from build123d import *

# Parameters (mm, degrees)
SKETCH1_W             = 152.4
SKETCH1_H             = 152.4
SKETCH1_W_2           = 127
SKETCH1_H_2           = 127
BOSS_EXTRUDE1_DEPTH   = 3.175
F_8_CLEARANCE_HOLE2_D = 4.4958
LPATTERN1_COUNT       = 2
LPATTERN1_PITCH       = 139.7
LPATTERN1_COUNT_DIR2  = 2
LPATTERN1_PITCH_DIR2  = 139.7


with BuildPart() as part:
    # Sketch1 → Boss-Extrude1 (new body)
    with BuildSketch(Plane.XY):
        with Locations((38.331291391, -35.471688742)):
            Rectangle(SKETCH1_W, SKETCH1_H)
        with Locations((38.331291391, -35.471688742)):
            Rectangle(SKETCH1_W_2, SKETCH1_H_2, mode=Mode.SUBTRACT)
    extrude(amount=BOSS_EXTRUDE1_DEPTH)

    # #8 Clearance Hole2 (through all)
    with Locations(Plane.XY.offset(3.175)):
        with Locations((-31.616116629, 34.273559139)):
            f_8_clearance_hole2 = Hole(F_8_CLEARANCE_HOLE2_D / 2)

    # LPattern1: 8 Clearance Hole2 2 × 2
    with Locations(*[(i * LPATTERN1_PITCH, -j * LPATTERN1_PITCH_DIR2, 0) for i in range(LPATTERN1_COUNT) for j in range(LPATTERN1_COUNT_DIR2) if (i, j) != (0, 0)]):
        add(f_8_clearance_hole2, mode=Mode.SUBTRACT)


solid = part.part
Here's how the part is built. I have some questions about the finished solid (model axes, mm). Coordinates: 2 decimals unless noted, no trailing zeros. Order: outer loops, then holes, each group sorted by start corner. A loop starts at its lowest first (then second) coordinate and runs counter-clockwise, first axis right, second up.
Item 1: If we section it at C-C on z = 1.95: List the corners of the cut face in (x, y) for me.
Result sheet:
outline: (-37.87, -111.67) - (114.53, -111.67) - (114.53, 40.73) - (-37.87, 40.73) - close; hole circle Ø4.5 at (-31.62, -105.43); hole circle Ø4.5 at (-31.62, 34.27); hole (-25.17, -98.97) - (101.83, -98.97) - (101.83, 28.03) - (-25.17, 28.03) - close; hole circle Ø4.5 at (108.08, -105.43); hole circle Ø4.5 at (108.08, 34.27)
Item 2: If we mould it in two halves opening along Y, with no side actions, what happens to faces 1 (the face through (-31.13, 32.08, 1.57)), 2 (the face through (105, -34, 3.175))? For each: +Y half, -Y half, draft (parallel to the pull), parting line (faces both ways), or undercut.
Result sheet:
face 1: undercut
face 2: draft
Item 3: For P1, Ø4, axis at x = 108.08, y = -105.43, coming from the +Z side; P2, Ø6, axis at x = -31.62, y = 34.27, coming from the +Z side (3 decimals), each with a flat end and sliding along its axis, tell me the tip position at first contact or that it passes through.
Result sheet:
P1: passes through
P2: stops at z = 3.175
Item 4: I need wall thicknesses on line 1 (X direction, y = -11, z = 1.2); line 2 (Y direction, x = 19.5, z = 1.5). Which ranges of each line are inside material? Lowest first, please.
Result sheet:
line 1: x = -37.87 to -25.17, 101.83 to 114.53
line 2: y = -111.67 to -98.97, 28.03 to 40.73
Item 5: If we section it at B-B on x = -9: List the corners of the cut face in (y, z) for me (3 decimals).
Result sheet:
outline: (-111.672, 0) - (-98.972, 0) - (-98.972, 3.175) - (-111.672, 3.175) - close; (28.028, 0) - (40.728, 0) - (40.728, 3.175) - (28.028, 3.175) - close
Item 6: If we section it at A-A on y = -57.5: List the corners of the cut face in (x, z) for me (3 decimals).
Result sheet:
outline: (-37.869, 0) - (-25.169, 0) - (-25.169, 3.175) - (-37.869, 3.175) - close; (101.831, 0) - (114.531, 0) - (114.531, 3.175) - (101.831, 3.175) - close
